from build123d import *

# Parameters (mm, degrees)
CROQUIS1_R              = 17.5
SALIENTE_EXTRUIR1_DEPTH = 6
CROQUIS2_R              = 2
CORTAR_EXTRUIR1_DEPTH   = 54.181293704
REDONDEO1_R             = 2


with BuildPart() as part:
    # Croquis1 → Saliente-Extruir1 (new, symmetric)
    with BuildSketch(Plane.XY):
        with BuildLine():
            Line((30, 0), (-30, 0))
            Line((-30, 0), (-30, 8))
            Line((-30, 8), (-22.5, 8))
            Line((-22.5, 8), (-22.5, 29))
            ThreePointArc((-22.5, 29), (0, 51.5), (22.5, 29))
            Line((22.5, 29), (22.5, 8))
            Line((22.5, 8), (30, 8))
            Line((30, 8), (30, 0))
        make_face()
        with Locations((0, 29)):
            Circle(CROQUIS1_R, mode=Mode.SUBTRACT)
    extrude(amount=SALIENTE_EXTRUIR1_DEPTH, both=True)

    # Croquis2 → Cortar-Extruir1 (cut, through all)
    with BuildSketch(Plane(origin=(0, 8, 0), x_dir=(1, 0, 0), z_dir=(0, 1, 0))):
        with Locations(Location((-26.25, 0, 0), (0, 0, 270))):
            Circle(CROQUIS2_R)
        with Locations(Location((26.25, 0, 0), (0, 0, 90))):
            Circle(CROQUIS2_R)
    extrude(amount=-CORTAR_EXTRUIR1_DEPTH, mode=Mode.SUBTRACT)

    # Redondeo1
    redondeo1_edges = [part.edges().sort_by_distance(p)[0] for p in [
        (30, 4, 6),
        (-30, 4, -6),
        (-30, 4, 6),
        (30, 4, -6),
    ]]
    fillet(redondeo1_edges, radius=REDONDEO1_R)


solid = part.part
Can you work these out from the model? Positions are in its coordinate system, mm. A direction names the side the tool comes from. Coordinates: 2 decimals unless noted, no trailing zeros. Loops run counter-clockwise (first coordinate to the right, second up) from the corner with the lowest first, then second, coordinate; pieces in that order, holes last. Notation, with made-up numbers: (-26.75, 52.25) - (32.25, 52.25) arc R34 cw to (32.25, 84.25) - close; hole circle Ø10 at (53, 46). An arc over 180 degrees is marked (long way). Put each result on its own line as item: value. Start each with the question number.
Item 1: If we mould it in two halves opening along X, with no side actions, what happens to faces 4 (the face through (24.5, 8, 1.4)), 5 (the face through (30, 4, 0)), 6 (the face through (-22.5, 18, 0)), 7 (the face through (-2.28, 46.35, -0.08))? For each: +X half, -X half, draft (parallel to the pull), parting line (faces both ways), or undercut.
Item 2: If I drill on line 1 along X through (y, z) = (6, 0); line 2 along Z through (x, y) = (26.25, 5.5); line 3 along Y through (x, z) = (0.5, 2.25), over which ranges is the centre line in solid material (lowest first)?
Item 3: Which directions (+Z, -Z, +X, -X, +Y, -Y) give clear straight access to the entire face, cutting with the end or side of a thin tool? Please do faces 1 (the face through (-29.4, 4.06, -5.43)), 2 (the face through (22.5, 19, 0)), 3 (the face through (-24.6, 8, 1.4)).
Item 4: Suppose I cut it at C-C (y = 25.5). Please give me the cut outline in (x, z).
Item 5: Suppose I cut it at D-D (z = 3). Please give me the cut outline in (x, y), and give its area (3 significant figures).
Item 6: Suppose I cut it at A-A (x = 0). Please give me the cut outline in (y, z), and give its area (3 significant figures).
Item 7: For pin 1 (3.5 mm diameter, centred on y = 20, z = -2, fed in from -X); pin 2 (1 mm diameter, centred on y = 38, z = 2.5, fed in from -X); pin 3 (3 mm diameter, centred on x = 0.5, z = 0, fed in from +Y), each with a flat end and sliding along its axis, tell me the tip position at first contact or that it passes through.
Item 8: Suppose I cut it at B-B (z = 0). Please give me the cut outline in (x, y), and give its area (3 significant figures).
Here are the results:
1. face 4: draft
1. face 5: +X half
1. face 6: -X half
1. face 7: undercut
2. line 1: -30 to -28.25, -24.25 to 24.25, 28.25 to 30
2. line 2: -6 to -2, 2 to 6
2. line 3: 0 to 11.51, 46.49 to 51.49
3. face 1: -Z, -X, +Y, -Y
3. face 2: +Z, -Z, +X, +Y
3. face 3: +Z, -Z, -X, +Y
4. outline: (-22.5, -6) - (-17.15, -6) - (-17.15, 6) - (-22.5, 6) - close; (17.15, -6) - (22.5, -6) - (22.5, 6) - (17.15, 6) - close
5. outline: (-30, 0) - (30, 0) - (30, 8) - (22.5, 8) - (22.5, 29) arc R22.5 ccw to (-22.5, 29) - (-22.5, 8) - (-30, 8) - close; hole circle Ø35 at (0, 29)
5. area: 1,260 mm²
6. outline: (0, -6) - (11.5, -6) - (11.5, 6) - (0, 6) - close; (46.5, -6) - (51.5, -6) - (51.5, 6) - (46.5, 6) - close
6. area: 198 mm²
7. pin 1: x = -22.5
7. pin 2: x = -20.83
7. pin 3: y = 51.5
8. outline: (-30, 0) - (-28.25, 0) - (-28.25, 8) - (-30, 8) - close; (-24.25, 0) - (24.25, 0) - (24.25, 8) - (22.5, 8) - (22.5, 29) arc R22.5 ccw to (-22.5, 29) - (-22.5, 8) - (-24.25, 8) - close; (28.25, 0) - (30, 0) - (30, 8) - (28.25, 8) - close; hole circle Ø35 at (0, 29)
8. area: 1,190 mm²
